Design review of the part built by this model. Coordinates are the model's own, in mm. A direction names the side the tool comes from. Coordinates: 2 decimals unless noted, no trailing zeros. Loops run counter-clockwise (first coordinate to the right, second up) from the corner with the lowest first, then second, coordinate; pieces in that order, holes last. Notation, with made-up numbers: (21.25, 87.25) -> (57.25, 87.25) arc R18 cw to (57.25, 113.25) -> close; hole circle Ø9 at (89, -30.5). An arc over 180 degrees is marked (long way). Answer in a Markdown table with one row per item.
```python
from build123d import *

# Parameters (mm, degrees)
F1_DEPTH  = 28
F2_W      = 211.909
F2_H      = 3
F3_DEPTH  = 15
F4_W      = 70
F4_H      = 3
F5_DEPTH  = 15
F7_DEPTH  = 3
F8_R      = 18.2181512029
F10_DEPTH = 3
F11_R     = 18.218
F13_DEPTH = 1
F15_DEPTH = 1


with BuildPart() as f1:
    # F0 (on Top) → F1 (new body)
    with BuildSketch(Plane.XY):
        with BuildLine():
            Line((23.2926856095, 0), (-81.7073143905, 0))
            Line((-81.7073143905, 0), (-81.7073143905, -15))
            Line((-81.7073143905, -15), (130.2926856095, -15))
            Line((130.2926856095, -15), (130.2926856095, 17))
            Line((130.2926856095, 17), (60.2926856095, 17))
            add(Edge.make_bspline(
                [(60.2926856095, 17), (47.0403235396, 17), (38.2657825675, 0), (23.2926856095, 0)],
                knots=[0, 0, 0, 0, 40.718546143, 40.718546143, 40.718546143, 40.718546143], degree=3))
        make_face()
    extrude(amount=-F1_DEPTH)

    # F2 (on face) → F3 (join)
    with BuildSketch(Plane(origin=(0, 0, 0), x_dir=(-1, 0, 0), z_dir=(0, 1, 0))):
        with Locations((-24.2471856095, -1.5)):
            Rectangle(F2_W, F2_H)
        with Locations((-24.2471856095, -26.5)):
            Rectangle(F2_W, F2_H)
    extrude(amount=F3_DEPTH)

    # F4 (on face) → F5 (join)
    with BuildSketch(Plane(origin=(0, 17, 0), x_dir=(-1, 0, 0), z_dir=(0, 1, 0))):
        with Locations((-95.2926856095, -26.5)):
            Rectangle(F4_W, F4_H)
        with Locations((-95.2926856095, -1.5)):
            Rectangle(F4_W, F4_H)
    extrude(amount=F5_DEPTH)

    # F6 (on face) → F7 (join)
    with BuildSketch(Plane.XY):
        Polygon((64.7905170918, 0), (60.2926856095, 32), (21.7418372631, 15), (26.0446537286, -15), align=None)
    extrude(amount=-F7_DEPTH)

    # F8
    f8_edges = [f1.edges().sort_by_distance(p)[0] for p in [
        (60.292686, 32, -1.5),
        (21.741837, 15, -1.5),
    ]]
    fillet(f8_edges, radius=F8_R)

    # F9 (on face) → F10 (join)
    with BuildSketch(Plane(origin=(0, 0, -28), x_dir=(1, 0, 0), z_dir=(0, 0, -1))):
        Polygon((24.2926856095, -15), (60.2926856095, -32), (60.2926856095, -17), (52.3001670697, -15), align=None)
    extrude(amount=-F10_DEPTH)

    # F11
    f11_edges = [f1.edges().sort_by_distance(p)[0] for p in [
        (60.292686, 32, -26.5),
        (24.292686, 15, -26.5),
    ]]
    fillet(f11_edges, radius=F11_R)

    # F12 (on face) → F13 (join)
    with BuildSketch(Plane.XY):
        with BuildLine():
            Line((130.2926856095, -15), (130.2926856095, 32))
            Line((130.2926856095, 32), (64.1312427554, 32))
            ThreePointArc((64.1312427554, 32), (60.3751547463, 31.6085937641), (56.7804614092, 30.4511933209))
            Line((56.7804614092, 30.4511933209), (25.2540614634, 16.5488066791))
            ThreePointArc((25.2540614634, 16.5488066791), (21.6593681263, 15.3914062359), (17.9032801172, 15))
            Line((17.9032801172, 15), (-81.7073143905, 15))
            Line((-81.7073143905, 15), (-81.7073143905, -15))
            Line((-81.7073143905, -15), (26.0446537286, -15))
            Line((26.0446537286, -15), (130.2926856095, -15))
        make_face()
    extrude(amount=F13_DEPTH)

    # F14 (on face) → F15 (join)
    with BuildSketch(Plane(origin=(0, 0, -28), x_dir=(1, 0, 0), z_dir=(0, 0, -1))):
        with BuildLine():
            ThreePointArc((20.2075043569, -15), (24.1936958703, -15.4414479941), (27.9867052288, -16.7443981536))
            Line((27.9867052288, -16.7443981536), (56.5986659901, -30.2556018464))
            ThreePointArc((56.5986659901, -30.2556018464), (60.3916753487, -31.5585520059), (64.3778668621, -32))
            Line((64.3778668621, -32), (130.2926856095, -32))
            Line((130.2926856095, -32), (130.2926856095, 15))
            Line((130.2926856095, 15), (-81.7073143905, 15))
            Line((-81.7073143905, 15), (-81.7073143905, -15))
            Line((-81.7073143905, -15), (20.2075043569, -15))
        make_face()
    extrude(amount=F15_DEPTH)


solid = f1.part
```
(1) For pin 1 (3 mm diameter, centred on x = -52, z = -26.5, fed in from +Y); pin 2 (6.5 mm diameter, centred on x = -8.5, z = -14, fed in from +Y); pin 3 (3 mm diameter, centred on y = 5.5, z = -13.5, fed in from -X), all flat-tipped, find the tip position at first contact; note any pin that passes through.
Evaluation:
| item | result |
|---|---|
| pin 1 | stops at y = 15 |
| pin 2 | stops at y = 0 |
| pin 3 | stops at x = 35.93 |
(2) Draft analysis for pull direction Z (two halves, no side actions). For faces 1 (the flat face through (26, 16, -3)), 2 (the flat face through (26, -15, -14)), 3 (the flat face through (23, 3, -29)), state which applies: pulls with the +Z half, pulls with the -Z half, needs draft (parallel to the pull), parting line crosses it, or undercut.
Evaluation:
| item | result |
|---|---|
| face 1 | undercut |
| face 2 | needs draft |
| face 3 | pulls with the -Z half |
(3) Take a section at C-C on x = 14. Give the boundary of the cut face in (y, z), and give its area (3 significant figures).
Evaluation:
| item | result |
|---|---|
| outline | (-15, -29) -> (15, -29) -> (15, -25) -> (0, -25) -> (0, -3) -> (15, -3) -> (15, 1) -> (-15, 1) -> close |
| area | 570 mm² |
(4) Tool access review of faces 4 (the flat face through (-28, 0, -14)), 5 (the flat face through (96, 17, -14)), 6 (the flat face through (98, 32, -1)), 7 (the flat face through (-31, 15, -27)), 8 (the flat face through (23, 4, 1)): name each direction out of +Z, -Z, +X, -X, +Y, -Y from which nothing blocks a thin tool from reaching the whole face with its end or side.
Evaluation:
| item | result |
|---|---|
| face 4 | -X, +Y |
| face 5 | +X, -X, +Y |
| face 6 | +Z, -Z, +X, -X, +Y |
| face 7 | +Z, -Z, -X, +Y |
| face 8 | +Z, +X, -X, +Y, -Y |
(5) Take a section at A-A on x = 80. Give the boundary of the cut face in (y, z).
Evaluation:
| item | result |
|---|---|
| outline | (-15, -29) -> (32, -29) -> (32, -25) -> (17, -25) -> (17, -3) -> (32, -3) -> (32, 1) -> (-15, 1) -> close |
(6) To check wall thickness, follow probe 1 along Z at (x, y) = (11, 14.5); probe 2 along Y at (x, z) = (-64.5, -9.5); probe 3 along Y at (x, z) = (5, -0.75). State the ranges of each line that lie inside material, in increasing order.
Evaluation:
| item | result |
|---|---|
| probe 1 | z = -29 to -25, -3 to 1 |
| probe 2 | y = -15 to 0 |
| probe 3 | y = -15 to 15 |
(7) Take a section at B-B on y = 22.5. Give the boundary of the cut face in (x, z).
Evaluation:
| item | result |
|---|---|
| outline | (38.75, -3) -> (130.29, -3) -> (130.29, 1) -> (38.75, 1) -> close; (40.18, -29) -> (130.29, -29) -> (130.29, -25) -> (40.18, -25) -> close |
